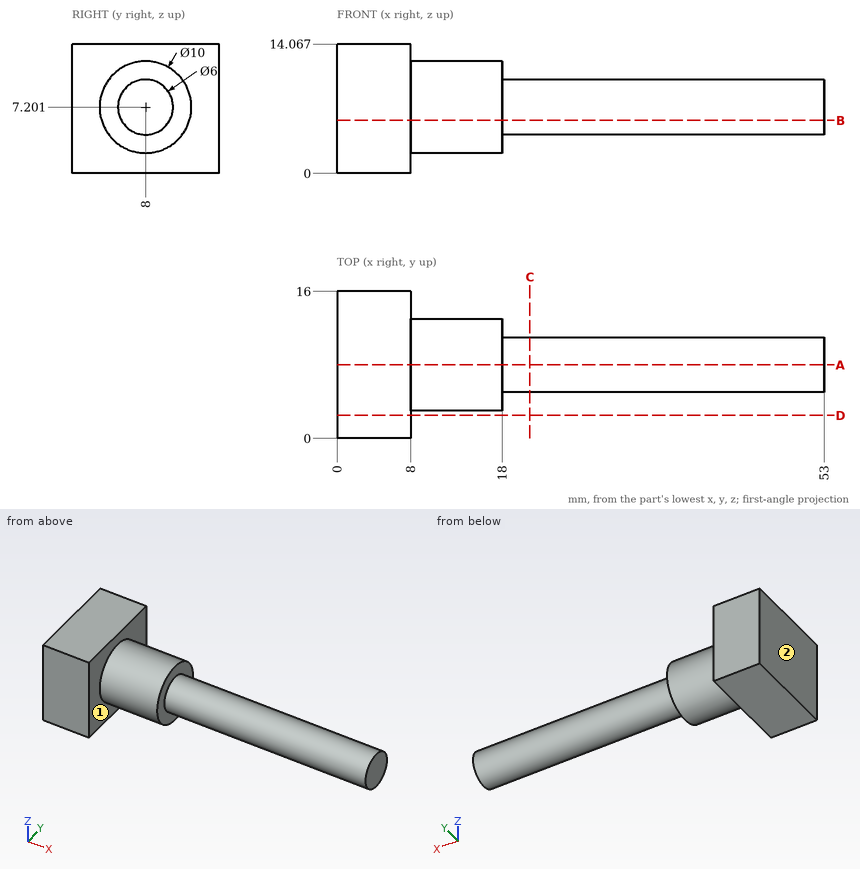
Verification items for this drawing (mm, ordinates from the low corner). A direction names the side the tool comes from. Give positions to 0.01 mm unless a question says otherwise; leave off trailing zeros. Write each loop counter-clockwise with the first axis right and the second up, starting at its lowest first coordinate (ties: lowest second). Pieces come first, ordered by that corner, then holes.
1) Section check C-C, the plane x = 21. Record the boundary of the cut face in (y, z).
2) Gauge pin test, flat ends, axial feed: pin 1 (4 mm diameter, centred on x = 38.5, z = 8.5, fed in from -Y); pin 2 (3 mm diameter, centred on x = 14, y = 11, fed in from -Z); pin 3 (5 mm diameter, centred on x = 21.5, y = 5.5, fed in from +Z); pin 4 (5 mm diameter, centred on y = 14, z = 9, fed in from -X). Record the tip position at first contact, or that the pin passes through.
3) Section check B-B, the plane z = 5.75. Record the boundary of the cut face in (x, y) (3 decimals).
4) Material ranges on L1, parallel to X at y = 13.5, z = 1.5; L2, parallel to Z at x = 15, y = 4; L3, parallel to Y at x = 38.5, z = 7.25, recorded low to high.
5) Section check A-A, the plane y = 8. Record the boundary of the cut face in (x, z), and give its area (3 significant figures).
6) Section check D-D, the plane y = 2.5. Record the boundary of the cut face in (x, z), and give its area (3 significant figures).
7) Access from +Z, -Z, +X, -X, +Y, -Y to the whole of each face (thin tool, end or side, straight path). Record for the marked faces 1 and 2.
Computed:
1. outline: circle Ø6 at (8, 7.2)
2. pin 1: stops at y = 5
2. pin 2: stops at z = 2.43
2. pin 3: stops at z = 10.2
2. pin 4: stops at x = 0
3. outline: (0, 0) - (8, 0) - (8, 3.215) - (18, 3.215) - (18, 5.374) - (53, 5.374) - (53, 10.626) - (18, 10.626) - (18, 12.785) - (8, 12.785) - (8, 16) - (0, 16) - close
4. L1: x = 0 to 8
4. L2: z = 4.2 to 10.2
4. L3: y = 5 to 11
5. outline: (0, 0) - (8, 0) - (8, 2.2) - (18, 2.2) - (18, 4.2) - (53, 4.2) - (53, 10.2) - (18, 10.2) - (18, 12.2) - (8, 12.2) - (8, 14.07) - (0, 14.07) - close
5. area: 423 mm2
6. outline: (0, 0) - (8, 0) - (8, 14.07) - (0, 14.07) - close
6. area: 113 mm2
7. face 1: +X
7. face 2: +Z, -Z, -X, +Y, -Y
